Source: CAD feature listing. Evaluate the final solid. Frame: model axes, mm. Coordinates: 2 decimals unless noted, no trailing zeros. Order: outer loops, then holes, each group sorted by start corner. A loop starts at its lowest first (then second) coordinate and runs counter-clockwise, first axis right, second up. Notation, with made-up numbers: (32.5, 59) - (51.5, 59) arc R32 cw to (51.5, 88) - close; hole circle Ø5 at (-10.5, 25). An arc over 180 degrees is marked (long way). One line per question, with ' | ' between items. Start each with the question number.
(1) Section C-C (z = 8.5). Return the cut outline in (x, y).
(2) Section A-A (x = -23.5). Return the cut outline in (y, z).
(3) Line query: line 1 along X through (y, z) = (3.65, 2); line 2 along Z through (x, y) = (-35.5, 0.75); line 3 along Z through (x, y) = (-24, 0.45). Output: solid intervals per line, ascending.
(4) Contact query for flat-ended pins moving along their axis: P1, Ø1.5, axis at x = 45.5, y = 3.5, coming from the +Z side; P2, Ø2.5, axis at x = 22.5, z = 27.67, coming from the +Y side; P3, Ø4.5, axis at x = -22.5, z = 27.67, coming from the +Y side; P4, Ø1, axis at y = 1, z = -24, coming from the +X side. Output: stop coordinate, or through.
(5) Section D-D (x = -36.5). Return the cut outline in (y, z).
(6) Section B-B (y = 1.4). Return the cut outline in (x, z), then the cut area to 3 significant figures.
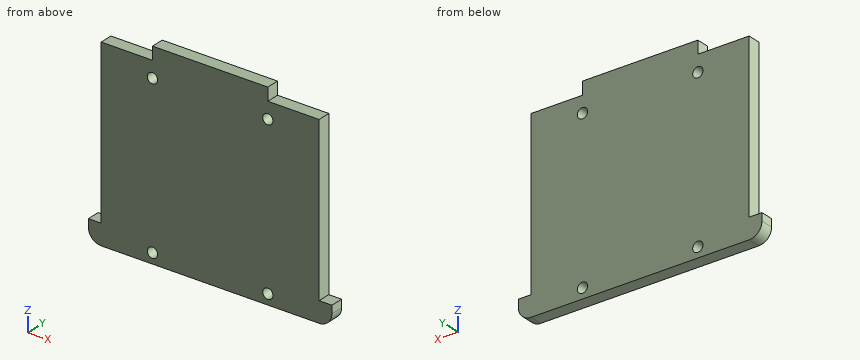
Autodesk Inventor part; units mm, degrees
ref_plane "YZ Plane" through (0, 0, 0) normal (1, 0, 0) x (0, 1, 0)
ref_plane "XZ Plane" through (0, 0, 0) normal (0, 1, 0) x (-1, 0, 0)
ref_plane "XY Plane" through (0, 0, 0) normal (0, 0, 1) x (1, 0, 0)
sketch "Sketch1" plane through (22.5, 0, 39.0178) normal (0, 1, 0) x (-1, 0, 0)
  line L0 (0.0005, -5) -> (0.0005, 0)
  line L1 (45.0005, 0) -> (0.0005, 0)
  line L2 (45.0005, 0) -> (45.0005, -5)
  circle A0 centre (-0.0005, -73) radius 2
  circle A1 centre (0, -11.3502) radius 2
  circle A2 centre (45, -11.3502) radius 2
  circle A3 centre (44.9998, -73) radius 2
  line L3 (-20, -5) -> (0.0005, -5)
  line L4 (45.0005, -5) -> (65.0008, -5)
  line L5 (-20, -69) -> (-25.0002, -69)
  line L6 (-25.0002, -69) -> (-25.0002, -72)
  arc A4 (-25.0002, -72) -> (-20, -77) centre (-20.0002, -72) ccw
  line L7 (-20, -77) -> (65, -77)
  arc A5 (65, -77) -> (70, -72) centre (65, -72) ccw
  line L8 (70, -72) -> (70, -69)
  line L9 (70, -69) -> (64.9998, -69)
  line L10 (-20, -69) -> (-20, -5)
  line L11 (64.9998, -69) -> (65.0008, -5)
  point P0 (-25.0005, -77)
  point P1 (11.4357, -9.3722)
  dimension "d5" = 4
  dimension "d1" = 4
  dimension "d0" = 4
extrude "Bottom Base" add sketch "Sketch1" along normal blind 5
properties part number "Bottom Base"
Response values:
1) outline: (-42.5, 0) - (42.5, 0) - (42.5, 5) - (-42.5, 5) - close
2) outline: (0, -37.98) - (5, -37.98) - (5, -35.71) - (0, -35.71) - close; (0, -32.25) - (5, -32.25) - (5, 25.94) - (0, 25.94) - close; (0, 29.4) - (5, 29.4) - (5, 34.02) - (0, 34.02) - close
3) line 1: x = -42.5 to 42.5 | line 2: z = -37.98 to 34.02 | line 3: z = -37.98 to -35.3, -32.66 to 26.34, 28.99 to 34.02
4) P1: stops at z = -29.98 | P2: passes through | P3: stops at y = 5 | P4: stops at x = 42.5
5) outline: (0, -37.98) - (5, -37.98) - (5, 34.02) - (0, 34.02) - close
6) outline: (-47.5, -32.98) arc R5 ccw to (-42.5, -37.98) - (42.5, -37.98) arc R5 ccw to (47.5, -32.98) - (47.5, -29.98) - (42.5, -29.98) - (42.5, 34.02) - (22.5, 34.02) - (22.5, 39.02) - (-22.5, 39.02) - (-22.5, 34.02) - (-42.5, 34.02) - (-42.5, -29.98) - (-47.5, -29.98) - close; hole circle Ø4 at (-22.5, -33.98); hole circle Ø4 at (-22.5, 27.67); hole circle Ø4 at (22.5, -33.98); hole circle Ø4 at (22.5, 27.67) | area: 6,360 mm²
